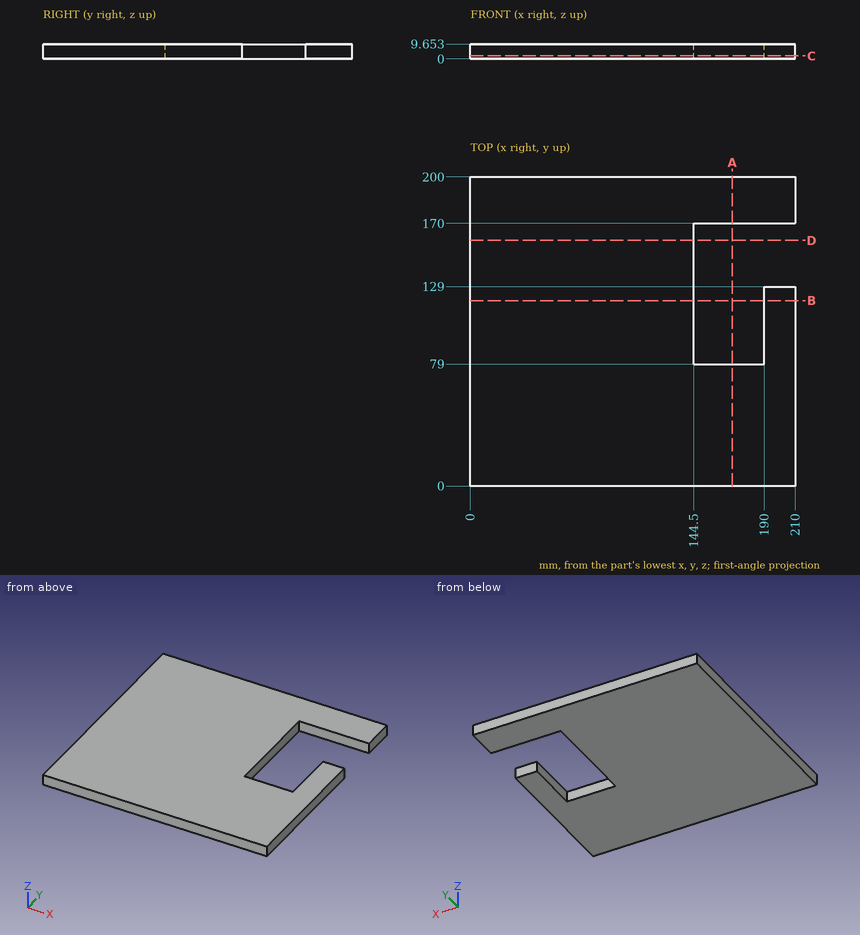
Check sheet for the drawn part. Datum: minimum x, y, z corner. Units: mm. Round coordinates to 2 decimals unless told otherwise and drop trailing zeros. Order: outer loops, then holes, each group sorted by start corner. A loop starts at its lowest first (then second) coordinate and runs counter-clockwise, first axis right, second up.
(1) Scan lines: probe 1 along X at (y, z) = (85, 1.5); probe 2 along Y at (x, z) = (153, 6); probe 3 along X at (y, z) = (150, 6.75). Record each from-to range of solid material in increasing order.
(2) Cross-section at B-B, the plane y = 120. Enter the section's corners in (x, z), and give its area (3 significant figures).
(3) Cross-section at D-D, the plane y = 159. Enter the section's corners in (x, z).
(4) Cross-section at A-A, the plane x = 169.5. Enter the section's corners in (y, z).
(5) Cross-section at C-C, the plane z = 2. Enter the section's corners in (x, y).
Check sheet entries:
1. probe 1: x = 0 to 144.5, 190 to 210
1. probe 2: y = 0 to 79, 170 to 200
1. probe 3: x = 0 to 144.5
2. outline: (0, 0) - (144.5, 0) - (144.5, 9.65) - (0, 9.65) - close; (190, 0) - (210, 0) - (210, 9.65) - (190, 9.65) - close
2. area: 1,590 mm2
3. outline: (0, 0) - (144.5, 0) - (144.5, 9.65) - (0, 9.65) - close
4. outline: (0, 0) - (79, 0) - (79, 9.65) - (0, 9.65) - close; (170, 0) - (200, 0) - (200, 9.65) - (170, 9.65) - close
5. outline: (0, 0) - (210, 0) - (210, 129) - (190, 129) - (190, 79) - (144.5, 79) - (144.5, 170) - (210, 170) - (210, 200) - (0, 200) - close
